Here's how the part is built. I have some questions about the finished solid (model axes, mm). A direction names the side the tool comes from. Give positions to 0.01 mm unless a question says otherwise; leave off trailing zeros. Loops run counter-clockwise (first coordinate to the right, second up) from the corner with the lowest first, then second, coordinate; pieces in that order, holes last. Notation, with made-up numbers: (27, 20) - (62, 20) arc R16 ccw to (62, 31) - close; hole circle Ø10 at (14, 86). An arc over 180 degrees is marked (long way). One line per item, written item: value. Start each with the question number.
```python
from build123d import *

# Parameters (mm, degrees)
BOSS_EXTRUDE1_DEPTH = 7
FILLET1_R           = 3.5
SKETCH2_R           = 2.2
SKETCH2_R_2         = 1.7
CUT_EXTRUDE1_DEPTH  = 47.376287044
FILLET2_SIZE        = 8
FILLET2_SIZE_2      = 2
FILLET3_START       = -1
FILLET3_DEPTH       = 9
FILLET3_2_DEPTH     = 7
SKETCH3_R           = 1.2
CUT_EXTRUDE2_DEPTH  = 47.376287108
SKETCH4_R           = 1.85
CUT_EXTRUDE3_DEPTH  = 2.4
CUT_EXTRUDE4_DEPTH  = 2.4


with BuildPart() as part:
    # Sketch1 → Boss-Extrude1 (new body)
    with BuildSketch(Plane(origin=(0, 0, 0), x_dir=(1, 0, 0), z_dir=(0, 1, 0))):
        Polygon((0, 0), (0, 40), (5, 40), (5, 25), (17.4, 25), (17.4, 40), (22.4, 40), (22.4, 0), (17.4, 0), (17.4, 15), (5, 15), (5, 0), align=None)
    extrude(amount=BOSS_EXTRUDE1_DEPTH)

    # Fillet1
    fillet1_edges = [part.edges().sort_by_distance(p)[0] for p in [
        (2.5, 0, -40),
        (2.5, 7, -40),
        (19.9, 0, -40),
        (19.9, 7, -40),
        (2.5, 0, 0),
        (2.5, 7, 0),
        (19.9, 0, 0),
        (19.9, 7, 0),
    ]]
    fillet(fillet1_edges, radius=FILLET1_R - 0.0001)  # a hair under: the kernel refuses the full size

    # Sketch2 → Cut-Extrude1 (cut, through all)
    with BuildSketch(Plane(origin=(22.4, 0, 0), x_dir=(0, 0, -1), z_dir=(1, 0, 0))):
        with Locations((3.5, 3.5)):
            Circle(SKETCH2_R)
        with Locations((36.5, 3.5)):
            Circle(SKETCH2_R_2)
    extrude(amount=-CUT_EXTRUDE1_DEPTH, mode=Mode.SUBTRACT)

    # Fillet2
    # a fillet whose section is not a circle: 8, 2 mm, written as the material it adds along each edge
    with BuildSketch(Plane(origin=(17.4, 0, -25), x_dir=(-1, 0, 0), z_dir=(0, 1, 0))) as fillet2_piece_1:
        with BuildLine():
            Bezier((FILLET2_SIZE, 0), (0, 0), (0, -FILLET2_SIZE_2), weights=[1, 0.707106781, 1])
            Line((0, -FILLET2_SIZE_2), (0, 0))
            Line((0, 0), (FILLET2_SIZE, 0))
        make_face()
    extrude(amount=7)

    # Fillet3: read off the stored shape, not the designer's step
    # Fillet3 outline → Fillet3 (cut)
    with BuildSketch(Plane(origin=(0, 0, 0), x_dir=(1.0, 3.4671016661374288e-12, 0), z_dir=(-3.4671016661374288e-12, 1.0, 2.5010475807975105e-12)).offset(FILLET3_START)):
        with BuildLine():
            add(Edge.make_bspline(
                [(15.582462981, 25.730719902), (12.297568617, 24.730707285), (9.28088208, 25)],
                knots=[0, 0, 0, 0.430571461, 0.430571461, 0.430571461], degree=2, weights=[1, 0.825748512, 0.80155246]))
            add(Edge.make_bspline(
                [(15.582462981, 25.730719902), (13.182155578, 25), (9.4, 25)],
                knots=[0.440891805, 0.440891805, 0.440891805, 1, 1, 1], degree=2, weights=[0.855599999, 0.836241001, 1]))
            Line((9.4, 25), (9.28088208, 25))
        make_face()
    extrude(amount=FILLET3_DEPTH, mode=Mode.SUBTRACT)

    # Fillet3 2 outline → Fillet3 2 (add)
    with BuildSketch(Plane(origin=(0, 0, 0), x_dir=(1.0, 3.4671016661374288e-12, 0), z_dir=(-3.4671016661374288e-12, 1.0, 2.5010475807975105e-12))):
        with BuildLine():
            Line((5, 25), (9.28088208, 25))
            add(Edge.make_bspline(
                [(9.28088208, 25), (5, 25.382144563), (5, 27.644025125)],
                knots=[0.430571461, 0.430571461, 0.430571461, 1, 1, 1], degree=2, weights=[0.80155246, 0.769553306, 1]))
            Line((5, 27.644025125), (5, 25))
        make_face()
        with BuildLine():
            Line((17.4, 15), (7.4, 15))
            add(Edge.make_bspline(
                [(7.4, 15), (17.4, 15), (17.4, 13)],
                knots=[0, 0, 0, 1, 1, 1], degree=2, weights=[1, 0.707106781, 1]))
            Line((17.4, 13), (17.4, 15))
        make_face()
    extrude(amount=FILLET3_2_DEPTH)

    # Sketch3 → Cut-Extrude2 (cut, through all)
    with BuildSketch(Plane.ZY):
        with Locations((-8, 3.5)):
            Circle(SKETCH3_R)
    extrude(amount=-CUT_EXTRUDE2_DEPTH, mode=Mode.SUBTRACT)

    # Sketch4 → Cut-Extrude3 (cut)
    with BuildSketch(Plane.ZY):
        with Locations((-8, 3.5)):
            Circle(SKETCH4_R)
    extrude(amount=-CUT_EXTRUDE3_DEPTH, mode=Mode.SUBTRACT)

    # Sketch5 → Cut-Extrude4 (cut)
    with BuildSketch(Plane(origin=(22.4, 0, 0), x_dir=(0, 0, -1), z_dir=(1, 0, 0))):
        Polygon((10.15, 4.741303079), (8, 5.982606158), (5.85, 4.741303079), (5.85, 2.258696921), (8, 1.017393842), (10.15, 2.258696921), align=None)
    extrude(amount=-CUT_EXTRUDE4_DEPTH, mode=Mode.SUBTRACT)


solid = part.part
```
(1) Please list where these lines run through material, in increasing order: probe 1 along Y at (x, z) = (21.2, -36.5); probe 2 along X at (y, z) = (5.5, -13); probe 3 along Z at (x, y) = (3.75, 2.25). Write a range as from..to.
(2) If we section it at B-B on z = -31: List the corners of the cut face in (x, y) for me.
(3) For faces 3 (the face through (5, 3, -33)), 4 (the face through (21.217, 1.647, -6.91)), 5 (the face through (5, 4.2, -9.3)), which set-ups out of +Z, -Z, +X, -X, +Y, -Y let a thin tool reach every point of the face, with its end or its side?
(4) If we section it at A-A on x = 2: Give the number of separate pieces and of enclosed holes in the cut face, plus the area to 3 significant figures.
(5) Will these pins go through, and if not, where does the flat tip stop? pin 1 (3 mm diameter, centred on y = 3.5, z = -8, fed in from +X); pin 2 (0.7 mm diameter, centred on x = 21, y = 3, fed in from -Z); pin 3 (1.8 mm diameter, centred on y = 3, z = -8, fed in from -X); pin 4 (2 mm diameter, centred on y = 3.5, z = -8, fed in from -X) (3 decimals).
(6) If we mould it in two halves opening along X, with no side actions, what happens to faces 1 (the face through (6, 3, -15)), 2 (the face through (2.46, 5.95, -1))? For each: pulls with the +X half, pulls with the -X half, needs draft (parallel to the pull), parting line crosses it, or undercut.
Found:
1. probe 1: 0..1.8, 5.2..7
1. probe 2: 0..5, 17.4..22.4
1. probe 3: -39.77..-37.65, -35.35..-5.31, -1.69..-0.23
2. outline: (0, 0) - (5, 0) - (5, 7) - (0, 7) - close; (17.4, 0) - (22.4, 0) - (22.4, 7) - (17.4, 7) - close
3. face 3: -Z, +Y, -Y
3. face 4: +X
3. face 5: +Z, +Y, -Y
4. separate pieces: 1
4. enclosed holes: 3
4. area: 234 mm^2
5. pin 1: x = 20
5. pin 2: z = -40
5. pin 3: x = 2.4
5. pin 4: through
6. face 1: undercut
6. face 2: needs draft
